Part model, mm, in its own coordinate system. Face numbers are marked on the shaded views. A direction names the side the tool comes from. Coordinates: 2 decimals unless noted, no trailing zeros. Loops run counter-clockwise (first coordinate to the right, second up) from the corner with the lowest first, then second, coordinate; pieces in that order, holes last. Notation, with made-up numbers: (74, 66.25) -> (122, 66.25) arc R16 cw to (122, 92.25) -> close; hole circle Ø7 at (60.5, -6). An arc over 180 degrees is marked (long way). One line per question, with ' | ' between items. Start each with the question number.
1) Cut at A-A (z = -8.5). List the corners of the cut face in (x, y).
2) Two-plate mould, pull along Y, no slides. Class the marked faces 1, 2, 3 and 4: released by +Y, released by -Y, zero draft, split by the parting line, or undercut.
3) 3-axis set-ups, long thin cutter, end or side, ignore diameter. For the marked faces 5, 6 and 7: which of +Z, -Z, +X, -X, +Y, -Y reach the whole face in a straight line?
4) Cut at C-C (z = -6). List the corners of the cut face in (x, y).
5) Cut at D-D (x = 0.5). List the corners of the cut face in (y, z).
6) Cut at B-B (y = 1.27). List the corners of the cut face in (x, z), plus the area to 3 significant figures.
7) Probe L1, parallel to Y at x = 1.2, z = -0.25; L2, parallel to Y at x = 0.95, z = -8.25; L3, parallel to Z at x = 1, y = 1.2. List the from-to ranges inside material, lowest first. Write a range as from..to.
from build123d import *

# Parameters (mm, degrees)
BOSS_EXTRUDE1_DEPTH = 1.6256


with BuildPart() as part:
    # Sketch1 → Boss-Extrude1 (new body)
    with BuildSketch(Plane(origin=(0, 0, 0), x_dir=(0, 0, -1), z_dir=(1, 0, 0))):
        with BuildLine():
            Line((0, 0), (6.35, 0))
            ThreePointArc((6.35, 0), (7.750762825, -0.753518252), (9.265164366, -0.267190977))
            ThreePointArc((9.265164366, -0.267190977), (9.317228392, 0.449340486), (8.600696929, 0.501404512))
            ThreePointArc((8.600696929, 0.501404512), (6.920229492, 1.27), (8.600696929, 2.038595488))
            ThreePointArc((8.600696929, 2.038595488), (9.317228392, 2.090659514), (9.265164366, 2.807190977))
            ThreePointArc((9.265164366, 2.807190977), (7.750762825, 3.293518252), (6.35, 2.54))
            Line((6.35, 2.54), (0, 2.54))
            Line((0, 2.54), (0, 0))
        make_face()
    extrude(amount=BOSS_EXTRUDE1_DEPTH)


solid = part.part
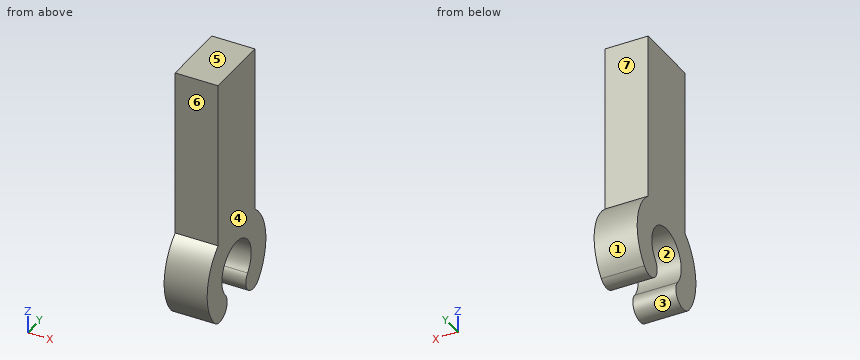
Reported:
1) outline: (0, -0.68) -> (1.63, -0.68) -> (1.63, 0.42) -> (0, 0.42) -> close; (0, 2.12) -> (1.63, 2.12) -> (1.63, 3.22) -> (0, 3.22) -> close
2) face 1: released by +Y | face 2: undercut | face 3: undercut | face 4: zero draft
3) face 5: +Z, +X, -X, +Y, -Y | face 6: +Z, +X, -X, -Y | face 7: +Z, +X, -X, +Y
4) outline: (0, 0) -> (1.63, 0) -> (1.63, 2.54) -> (0, 2.54) -> close
5) outline: (-0.27, -9.27) arc R0.51 ccw to (0.5, -8.6) arc R1.02 cw (long way) to (2.04, -8.6) arc R0.51 ccw to (2.81, -9.27) arc R2.03 ccw to (2.54, -6.35) -> (2.54, 0) -> (0, 0) -> (0, -6.35) arc R2.03 ccw to start
6) outline: (0, -6.92) -> (1.63, -6.92) -> (1.63, 0) -> (0, 0) -> close | area: 11.2 mm²
7) L1: y = 0..2.54 | L2: y = -0.74..0.3, 2.24..3.28 | L3: z = -6.92..0
